Read the model definition and answer for the solid it produces. Units are mm, in the model's axes. Face numbers are marked on the shaded views. A direction names the side the tool comes from. Coordinates: 2 decimals unless noted, no trailing zeros. Write each loop counter-clockwise with the first axis right and the second up, starting at its lowest first coordinate (ties: lowest second). Pieces come first, ordered by that corner, then holes.
1) The part is cut by section D-D (y = -50). Determine the outline of the cut face in (x, z) (3 decimals).
2) Determine the mould class of the marked faces 3, 4 and 5 for opening direction Y: +Y half, -Y half, draft (parallel to the pull), parting line (faces both ways), or undercut.
3) Each of these flat-tipped pins is pushed along its axis until it touches: pin 1 Ø3 at (x, y) = (-14.07, -12.11) entering from -Z; pin 2 Ø4.5 at (x, y) = (-14.07, 13.89) entering from +Z; pin 3 Ø3 at (x, y) = (14.5, 37) entering from -Z. Where does it stop, or does it pass through?
4) Find the intervals of material crossed by line 1 (Y direction, x = 0, z = 21); line 2 (Y direction, x = 1.5, z = 23); line 3 (X direction, y = -50, z = 45) (3 decimals), in increasing order.
5) Which of the six approach directions +Z, -Z, +X, -X, +Y, -Y give full straight-line access (tool end or side, diameter ignored) to the marked faces 1 and 2?
6) The part is cut by section B-B (y = -80). Determine the outline of the cut face in (x, z) (3 decimals), then the cut area to 3 significant figures.
7) The part is cut by section A-A (x = 0). Determine the outline of the cut face in (y, z).
8) The part is cut by section C-C (z = 28). Determine the outline of the cut face in (x, y) (3 decimals).
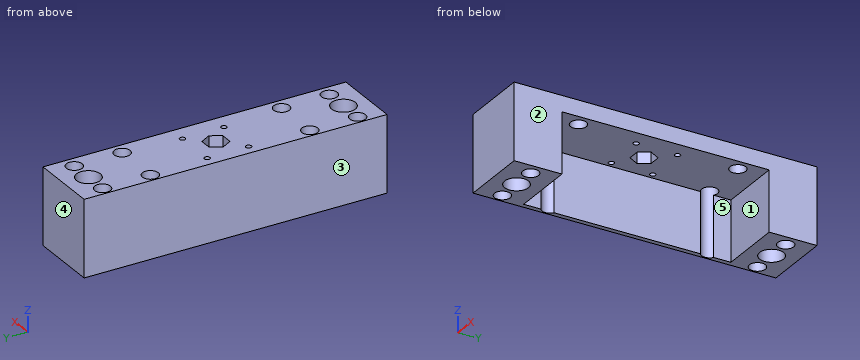
from build123d import *

# Parameters (mm, degrees)
F0_R     = 5
F0_R_2   = 7.5
F0_R_3   = 1.75
F2_DEPTH = 48
F3_DEPTH = 48
F4_W     = 130
F4_H     = 38
F5_DEPTH = 48.3
F6_W     = 8
F6_H     = 190
F7_DEPTH = 50


with BuildPart() as f2:
    # F0 (on Top) → F2 (new body)
    with BuildSketch(Plane.XY):
        Polygon((-20.6482383256, 95), (-20.6482383256, 17.5979303911), (-20.6482383256, 0), (-20.6482383256, -17.5979303911), (-20.6482383256, -95), (30.6482383256, -95), (30.6482383256, 0), (30.6482383256, 95), align=None)
        with Locations((-14.875, -80)):
            Circle(F0_R, mode=Mode.SUBTRACT)
        with Locations((-14.875, -50)):
            Circle(F0_R, mode=Mode.SUBTRACT)
        with Locations((0, -80)):
            Circle(F0_R_2, mode=Mode.SUBTRACT)
        with Locations((-14.0701553242, -12.1067194764)):
            Circle(F0_R_3, mode=Mode.SUBTRACT)
        with Locations((14.875, -80)):
            Circle(F0_R, mode=Mode.SUBTRACT)
        with Locations((14.875, -50)):
            Circle(F0_R, mode=Mode.SUBTRACT)
        with Locations((11.9298446758, -12.1067194764)):
            Circle(F0_R_3, mode=Mode.SUBTRACT)
        with Locations((-14.0701553242, 13.8932805236)):
            Circle(F0_R_3, mode=Mode.SUBTRACT)
        with Locations((-14.875, 50)):
            Circle(F0_R, mode=Mode.SUBTRACT)
        with Locations((-14.875, 80)):
            Circle(F0_R, mode=Mode.SUBTRACT)
        with Locations((0, 80)):
            Circle(F0_R_2, mode=Mode.SUBTRACT)
        with Locations((11.9298446758, 13.8932805236)):
            Circle(F0_R_3, mode=Mode.SUBTRACT)
        with Locations((14.875, 50)):
            Circle(F0_R, mode=Mode.SUBTRACT)
        with Locations((14.875, 80)):
            Circle(F0_R, mode=Mode.SUBTRACT)
    extrude(amount=F2_DEPTH)

    # F1 (on face) → F3 (cut)
    with BuildSketch(Plane.XY):
        Polygon((3.7816442632, 6.55), (-3.7816442632, 6.55), (-7.5632885264, 0), (-3.7816442632, -6.55), (3.7816442632, -6.55), (7.5632885264, 0), align=None)
    extrude(amount=F3_DEPTH, mode=Mode.SUBTRACT)

    # F4 (on face) → F5 (cut)
    with BuildSketch(Plane.YZ.offset(30.6482383256)):
        with Locations((0, 19)):
            Rectangle(F4_W, F4_H)
    extrude(amount=-F5_DEPTH, mode=Mode.SUBTRACT)

    # F6 (on face) → F7 (cut)
    with BuildSketch(Plane.XY.offset(48)):
        with Locations((26.6482383256, 0)):
            Rectangle(F6_W, F6_H)
    extrude(amount=-F7_DEPTH, mode=Mode.SUBTRACT)


solid = f2.part
Reported:
1. outline: (-20.648, 0) - (-19.875, 0) - (-19.875, 48) - (-20.648, 48) - close; (-9.875, 38) - (9.875, 38) - (9.875, 48) - (-9.875, 48) - close; (19.875, 38) - (22.648, 38) - (22.648, 48) - (19.875, 48) - close
2. face 3: draft
2. face 4: +Y half
2. face 5: undercut
3. pin 1: passes through
3. pin 2: stops at z = 48
3. pin 3: stops at z = 38
4. line 1: y = -95 to -87.5, -72.5 to -65, 65 to 72.5, 87.5 to 95
4. line 2: y = -95 to -87.35, -72.65 to -65, 65 to 72.65, 87.35 to 95
4. line 3: x = -20.648 to -19.875, -9.875 to 9.875, 19.875 to 22.648
5. face 1: -Z, +X
5. face 2: +Z, -Z, +X, +Y, -Y
6. outline: (-20.648, 0) - (-19.875, 0) - (-19.875, 48) - (-20.648, 48) - close; (-9.875, 0) - (-7.5, 0) - (-7.5, 48) - (-9.875, 48) - close; (7.5, 0) - (9.875, 0) - (9.875, 48) - (7.5, 48) - close; (19.875, 0) - (22.648, 0) - (22.648, 48) - (19.875, 48) - close
6. area: 398 mm2
7. outline: (-95, 0) - (-87.5, 0) - (-87.5, 48) - (-95, 48) - close; (-72.5, 0) - (-65, 0) - (-65, 38) - (-6.55, 38) - (-6.55, 48) - (-72.5, 48) - close; (6.55, 38) - (65, 38) - (65, 0) - (72.5, 0) - (72.5, 48) - (6.55, 48) - close; (87.5, 0) - (95, 0) - (95, 48) - (87.5, 48) - close
8. outline: (-20.648, -95) - (22.648, -95) - (22.648, -65) - (-17.652, -65) - (-17.652, -54.158) arc R5 cw to (-17.652, -45.842) - (-17.652, 45.842) arc R5 cw to (-17.652, 54.158) - (-17.652, 65) - (22.648, 65) - (22.648, 95) - (-20.648, 95) - close; hole circle Ø10 at (-14.875, -80); hole circle Ø10 at (-14.875, 80); hole circle Ø15 at (0, -80); hole circle Ø15 at (0, 80); hole circle Ø10 at (14.875, -80); hole circle Ø10 at (14.875, 80)
